CAD build for the part. Positions are in the model's coordinates, mm. Round coordinates to 2 decimals unless told otherwise and drop trailing zeros. Loops run counter-clockwise (first coordinate to the right, second up) from the corner with the lowest first, then second, coordinate; pieces in that order, holes last. Notation, with made-up numbers: (74, 63) -> (114, 63) arc R22 cw to (114, 92) -> close; hole circle Ø7 at (49, -15). An arc over 180 degrees is marked (long way). Answer as CSV lines item,"result".
Autodesk Inventor part; units mm, degrees
ref_plane "Arbeitsebene1" through (0, 0, 3.8) normal (0, 0, 1) x (1, 0, 0)
ref_plane "Arbeitsebene2" through (0, 0, 0) normal (1, 0, 0) x (0, 1, 0)
ref_plane "Arbeitsebene3" through (0, 0, 2.4) normal (0, 0, -1) x (-1, 0, 0)
sketch "Skizze3" plane through (0, 0, 0) normal (0, 0, 1) x (1, 0, 0)
  circle A0 centre (0, 0) radius 1.25
  dimension "d0" = 2.5
extrude "Extrusion1" add sketch "Skizze3" along normal blind 4.8
ref_plane "Arbeitsebene1" through (0, 0, 3.8) normal (0, 0, 1) x (1, 0, 0)
split_face "Trennen1"
ref_plane "Arbeitsebene2" through (0, 0, 0) normal (1, 0, 0) x (0, 1, 0)
sketch "Skizze6" plane through (0, 0, 0) normal (1, 0, 0) x (0, 1, 0)
  line L0 (0, 4.8) -> (0, 7.23)
  arc A0 (0, 7.23) -> (-0.25, 7.48) centre (-0.25, 7.23) ccw
  line L1 (-0.25, 7.23) -> (-0.25, 7.48) construction
  line L2 (-0.25, 7.23) -> (0, 7.23) construction
  line L3 (-0.25, 7.48) -> (-4.25, 7.48)
  line L4 (1.25, 4.8) -> (-1.25, 4.8)
  line L5 (1.25, 4.8) -> (1.25, 3.8)
  line L6 (1.25, 3.8) -> (1.25, 0)
  line L7 (1.25, 0) -> (-1.25, 0)
  line L8 (-1.25, 0) -> (-1.25, 3.8)
  line L9 (-1.25, 3.8) -> (-1.25, 4.8)
  line L10 (-1.25, 4.8) -> (1.25, 4.8)
  line L11 (-1.25, 3.8) -> (-1.25, 4.8)
  point P0 (0, 0)
  dimension "d7" = 90
  dimension "d9" = 2.43
  dimension "d10" = 4
  dimension "d13" = 0.25
  dimension "d20" = 0.25
  dimension "d21" = 1.25
sketch "Skizze4" plane through (0, 0, 4.8) normal (0, 0, 1) x (1, 0, 0)
  circle A0 centre (0, 0) radius 0.25
  dimension "d4" = 0.5
sweep "Sweeping1" add profiles "Skizze4" path "Skizze6" path curves L0 A0 L3
ref_plane "Arbeitsebene3" through (0, 0, 2.4) normal (0, 0, -1) x (-1, 0, 0)
mirror "Spiegeln1" about plane through (0, 0, 2.4) normal (0, 0, -1) of "Sweeping1"
properties part number "Diod1e"
Q1. Slice it at C-C, the plane z = 6.25. Give the cut face in (x, y).
Results:
outline,"circle Ø0.5 at (0, 0)"
Q2. Slice it at B-B, the plane x = -0.35. Give the cut face in (y, z).
Results:
outline,"(-1.2, 0) -> (1.2, 0) -> (1.2, 4.8) -> (-1.2, 4.8) -> close"
Q3. Slice it at D-D, the plane y = 0.8. Give the cut face in (x, z), and give its area (3 significant figures).
Results:
outline,"(-0.96, 0) -> (0.96, 0) -> (0.96, 4.8) -> (-0.96, 4.8) -> close"
area,"9.22 mm2"
Q4. Drop flat-ended pins along their axis: pin 1 Ø2 at (y, z) = (-2, 3.5) entering from +X; pin 2 Ø1.2 at (x, y) = (-0.5, 0.5) entering from -Z. Give the stop position or say it passes through.
Results:
pin 1,"x = 0.75"
pin 2,"z = -2.8"
Q5. Probe L1, parallel to Z at x = 1.15, y = 0.4; L2, parallel to Z at x = 0, y = -2.95; L3, parallel to Z at x = 0.15, y = -2.1. List the from-to ranges inside material, lowest first. Write a range as [from, to].
Results:
L1,"[0, 4.8]"
L2,"[-2.93, -2.43], [7.23, 7.73]"
L3,"[-2.88, -2.48], [7.28, 7.68]"
Q6. Slice it at A-A, the plane y = -2.2. Give the cut face in (x, z), and give its area (3 significant figures).
Results:
outline,"circle Ø0.5 at (0, -2.68); circle Ø0.5 at (0, 7.48)"
area,"0.393 mm2"
